```python
from build123d import *

# Parameters (mm, degrees)
SKETCH_1_R          = 35.5
EXTRUDE_1_DEPTH     = 1.5
SKETCH_2_R          = 3.5
CUT_EXTRUDE_1_DEPTH = 2
SKETCH_3_R          = 1.5
CUT_EXTRUDE_2_DEPTH = 2
SKETCH_5_R          = 1.5
CUT_EXTRUDE_3_DEPTH = 2


with BuildPart() as part:
    # 草图1 → 凸台-拉伸1 (new body)
    with BuildSketch(Plane.XY):
        Circle(SKETCH_1_R)
    extrude(amount=EXTRUDE_1_DEPTH)

    # 草图2 → 切除-拉伸1 (cut)
    with BuildSketch(Plane.XY.offset(1.5)):
        Circle(SKETCH_2_R)
    extrude(amount=-CUT_EXTRUDE_1_DEPTH, mode=Mode.SUBTRACT)

    # 草图3 → 切除-拉伸2 (cut)
    with BuildSketch(Plane.XY.offset(1.5)):
        with Locations((0, 7)):
            Circle(SKETCH_3_R)
        with Locations((7, 0)):
            Circle(SKETCH_3_R)
        with Locations((0, -7)):
            Circle(SKETCH_3_R)
        with Locations((-7, 0)):
            Circle(SKETCH_3_R)
    extrude(amount=-CUT_EXTRUDE_2_DEPTH, mode=Mode.SUBTRACT)

    # 草图5 → 切除-拉伸3 (cut)
    with BuildSketch(Plane.XY.offset(1.5)):
        with Locations((-31, 0)):
            Circle(SKETCH_5_R)
        with Locations((15.5, 26.846787517)):
            Circle(SKETCH_5_R)
        with Locations((15.5, -26.846787517)):
            Circle(SKETCH_5_R)
    extrude(amount=-CUT_EXTRUDE_3_DEPTH, mode=Mode.SUBTRACT)


solid = part.part
```
Geometry: final body of the model. Coordinates: model frame, mm. Give positions to 0.01 mm unless a question says otherwise; leave off trailing zeros. Write each loop counter-clockwise with the first axis right and the second up, starting at its lowest first coordinate (ties: lowest second). Pieces come first, ordered by that corner, then holes.
1. Section query C-C, the plane z = 1.05. Count the separate pieces of the cut face and the enclosed holes in it, then the cut area to 3 significant figures.
2. Section query B-B, the plane y = 0. Return loops of the section in (x, z).
3. Section query D-D, the plane y = -23.5. Return loops of the section in (x, z).
4. Draft query along X for faces 1 (the cylindrical face through (-7.696, -34.656, 0.74)), 2 (the cylindrical face through (-8.5, 0.07, 0.76)), 3 (the flat face through (7, -7, 0)). Return one class per face: released by +X, released by -X, zero draft, split by the parting line, or undercut.
5. Line query: probe 1 along Y at (x, z) = (0, 1); probe 2 along Y at (x, z) = (15.5, 0.95); probe 3 along X at (y, z) = (-1, 1.2). Output: solid intervals per line, ascending.
6. Section query A-A, the plane x = 0. Return loops of the section in (y, z).
7. Pin query (flat end, axial travel): P1, Ø1.8, axis at x = 15.5, y = -26.85, coming from the +Z side. Return the tip coordinate at first contact, or that it passes through.
Computed:
1. separate pieces: 1
1. enclosed holes: 8
1. area: 3,870 mm2
2. outline: (-35.5, 0) - (-32.5, 0) - (-32.5, 1.5) - (-35.5, 1.5) - close; (-29.5, 0) - (-8.5, 0) - (-8.5, 1.5) - (-29.5, 1.5) - close; (-5.5, 0) - (-3.5, 0) - (-3.5, 1.5) - (-5.5, 1.5) - close; (3.5, 0) - (5.5, 0) - (5.5, 1.5) - (3.5, 1.5) - close; (8.5, 0) - (35.5, 0) - (35.5, 1.5) - (8.5, 1.5) - close
3. outline: (-26.61, 0) - (26.61, 0) - (26.61, 1.5) - (-26.61, 1.5) - close
4. face 1: split by the parting line
4. face 2: undercut
4. face 3: zero draft
5. probe 1: y = -35.5 to -8.5, -5.5 to -3.5, 3.5 to 5.5, 8.5 to 35.5
5. probe 2: y = -31.94 to -28.35, -25.35 to 25.35, 28.35 to 31.94
5. probe 3: x = -35.49 to -32.12, -29.88 to -8.12, -5.88 to -3.35, 3.35 to 5.88, 8.12 to 35.49
6. outline: (-35.5, 0) - (-8.5, 0) - (-8.5, 1.5) - (-35.5, 1.5) - close; (-5.5, 0) - (-3.5, 0) - (-3.5, 1.5) - (-5.5, 1.5) - close; (3.5, 0) - (5.5, 0) - (5.5, 1.5) - (3.5, 1.5) - close; (8.5, 0) - (35.5, 0) - (35.5, 1.5) - (8.5, 1.5) - close
7. P1: passes through
